Source: three-view drawing plus pictorial views. Frame: mm from the lowest corner of the part. Give positions to 0.01 mm unless a question says otherwise; leave off trailing zeros. Write each loop counter-clockwise with the first axis right and the second up, starting at its lowest first coordinate (ties: lowest second). Pieces come first, ordered by that corner, then holes.
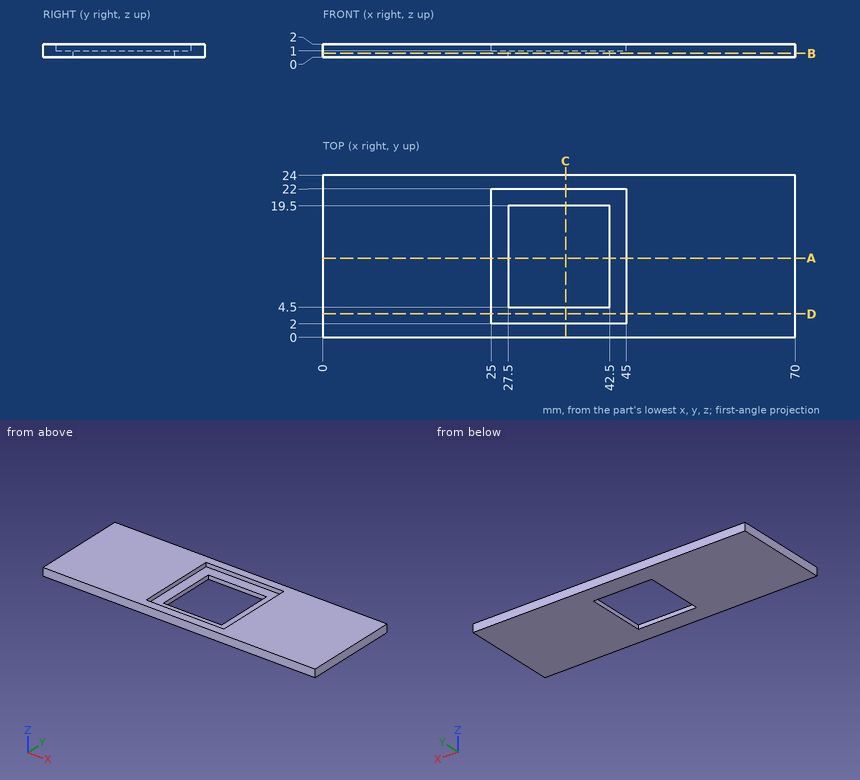
Q1. Ray query, line 1 along X through (y, z) = (3, 1.8); line 2 along X through (y, z) = (11, 0.7); line 3 along Y through (x, z) = (41, 1.4). Return the intervals inside material, ascending.
Filled sheet:
line 1: x = 0 to 25, 45 to 70
line 2: x = 0 to 27.5, 42.5 to 70
line 3: y = 0 to 2, 22 to 24
Q2. Section C-C on x = 36. Output: boundary loops of the cut face in (y, z), plus the area to 3 significant figures.
Filled sheet:
outline: (0, 0) - (4.5, 0) - (4.5, 1) - (2, 1) - (2, 2) - (0, 2) - close; (19.5, 0) - (24, 0) - (24, 2) - (22, 2) - (22, 1) - (19.5, 1) - close
area: 13.0 mm2
Q3. Section B-B on z = 0.6. Output: boundary loops of the cut face in (x, y), plus the area to 4 significant figures.
Filled sheet:
outline: (0, 0) - (70, 0) - (70, 24) - (0, 24) - close; hole (27.5, 4.5) - (42.5, 4.5) - (42.5, 19.5) - (27.5, 19.5) - close
area: 1,455 mm2
Q4. Section D-D on y = 3.5. Output: boundary loops of the cut face in (x, z).
Filled sheet:
outline: (0, 0) - (70, 0) - (70, 2) - (45, 2) - (45, 1) - (25, 1) - (25, 2) - (0, 2) - close
Q5. Pin query (flat end, axial travel): P1, Ø2, axis at x = 34, y = 19.5, coming from the +Z side. Return the tip coordinate at first contact, or that it passes through.
Filled sheet:
P1: stops at z = 1
Q6. Section A-A on y = 11.75. Output: boundary loops of the cut face in (x, z).
Filled sheet:
outline: (0, 0) - (27.5, 0) - (27.5, 1) - (25, 1) - (25, 2) - (0, 2) - close; (42.5, 0) - (70, 0) - (70, 2) - (45, 2) - (45, 1) - (42.5, 1) - close
